The drawing under review shows one solid part. Ordinate dimensions are in mm from its lowest x, y, z. Coordinates: 2 decimals unless noted, no trailing zeros. Loops run counter-clockwise (first coordinate to the right, second up) from the corner with the lowest first, then second, coordinate; pieces in that order, holes last. Notation, with made-up numbers: (9, -11) - (29, -11) arc R18 cw to (29, 19) - close; hole circle Ø8 at (-13, -22.75). An arc over 180 degrees is marked (long way). Use one line per item in the form item = value. Start each with the question number.
1. Add section A-A on y = 44.7. Give the boundary of the cut face in (x, z), and give its area (3 significant figures).
2. Add section C-C on z = 4.25. Give the boundary of the cut face in (x, y).
3. Add section B-B on x = 158.5. Give the boundary of the cut face in (y, z).
4. To check wall thickness, follow probe 1 along Y at (x, z) = (94.5, 7); probe 2 along X at (y, z) = (44.7, 2.75); probe 3 along X at (y, z) = (29, 1.5). State the ranges of each line that lie inside material, in increasing order.
5. For pin 1 Ø2 at (x, y) = (57, 36.5) entering from -Z, flat-tipped, find the tip position at first contact; note if it passes through.
6. Add section D-D on y = 25.5. Give the boundary of the cut face in (x, z).
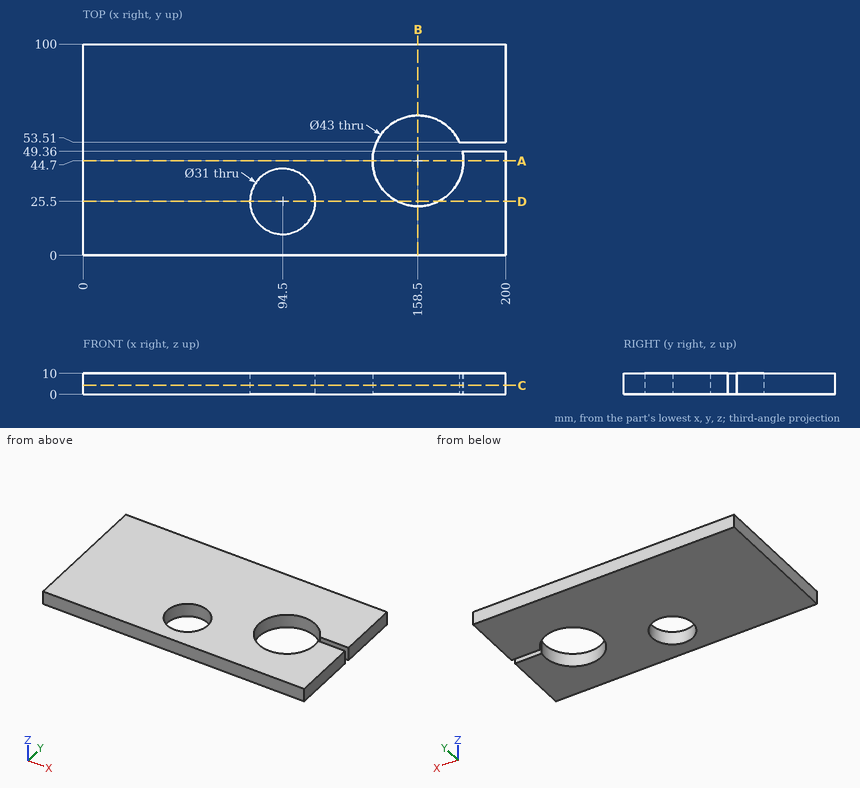
Conclusion:
q1.outline = (0, 0) - (137, 0) - (137, 10) - (0, 10) - close; (180, 0) - (200, 0) - (200, 10) - (180, 10) - close
q1.area = 1,570 mm^2
q2.outline = (0, 0) - (200, 0) - (200, 49.36) - (179.49, 49.36) arc R21.5 cw (long way) to (178.11, 53.51) - (200, 53.51) - (200, 100) - (0, 100) - close; hole circle Ø31 at (94.5, 25.5)
q3.outline = (0, 0) - (23.2, 0) - (23.2, 10) - (0, 10) - close; (66.2, 0) - (100, 0) - (100, 10) - (66.2, 10) - close
q4.probe_1 = 0 to 10, 41 to 100
q4.probe_2 = 0 to 137, 180 to 200
q4.probe_3 = 0 to 79.4, 109.6 to 143.81, 173.19 to 200
q5.pin_1 = 0
q6.outline = (0, 0) - (79, 0) - (79, 10) - (0, 10) - close; (110, 0) - (148.82, 0) - (148.82, 10) - (110, 10) - close; (168.18, 0) - (200, 0) - (200, 10) - (168.18, 10) - close
